Autodesk Inventor part; units mm, degrees
ref_plane "YZ Plane" through (0, 0, 0) normal (1, 0, 0) x (0, 1, 0)
ref_plane "XZ Plane" through (0, 0, 0) normal (0, 1, 0) x (-1, 0, 0)
ref_plane "XY Plane" through (0, 0, 0) normal (0, 0, 1) x (1, 0, 0)
sketch "Sketch1" plane through (0, 0, 0) normal (0, 1, 0) x (-1, 0, 0)
  line L0 (-3.8, -5.08) -> (100.076, -5.08)
  line L1 (100.076, -5.08) -> (100.076, 66.04)
  line L2 (100.076, 66.04) -> (-3.8, 66.04)
  line L3 (-3.8, 66.04) -> (-3.8, -5.08)
  circle A0 centre (11.176, 62.23) radius 1.75
  circle A1 centre (96.266, 62.23) radius 1.75
  circle A2 centre (96.266, 4.318) radius 1.75
  circle A3 centre (22.86, 4.318) radius 1.75
  line L4 (10.922, -14.9293) -> (10.922, -25.1011) construction
  point P0 (0, 0)
  dimension "d1" = 3.8
  dimension "d2" = 5.08
  dimension "d3" = 100.076
  dimension "d4" = 66.04
  dimension "d5" = 22.86
  dimension "d6" = 4.318
  dimension "d7" = 3.5
  dimension "d8" = 96.266
  dimension "d9" = 4.318
  dimension "d10" = 3.5
  dimension "d11" = 62.23
  dimension "d12" = 11.176
  dimension "d13" = 3.5
  dimension "d14" = 3.5
  dimension "d15" = 10.922
  dimension "d16" = 11.938
extrude "Extrusion1" add sketch "Sketch1" along normal blind 2
sketch "Sketch2" plane through (0, 2, 0) normal (0, 1, 0) x (1, 0, 0)
  circle A0 centre (-22.86, -4.318) radius 1.75
  line L0 (-16.922, 10.48) -> (-4.922, 10.48)
  line L1 (-4.922, 10.48) -> (-4.922, -4.318)
  line L2 (-4.922, -4.318) -> (-16.922, -4.318)
  line L3 (-16.922, -4.318) -> (-16.922, 10.48)
  line L4 (-10.922, -7.2674) -> (-10.922, -16.4399) construction
  line L5 (3.8, 5.08) -> (-100.076, 5.08)
  point P0 (0, 0)
  dimension "d20" = 11.938
  dimension "d21" = 6
  dimension "d22" = 12
  dimension "d25" = 5.4
extrude "Extrusion2" add sketch "Sketch2" along normal blind 12 contours L0 L1 L5 L3 | L5 L1 L2 L3
properties part number "printrboard"
Check sheet for the modelled part. Datum: model origin and axes. Units: mm. A direction names the side the tool comes from. Round coordinates to 2 decimals unless told otherwise and drop trailing zeros. Order: outer loops, then holes, each group sorted by start corner. A loop starts at its lowest first (then second) coordinate and runs counter-clockwise, first axis right, second up. Notation, with made-up numbers: (-18, 65) -> (-13, 65) arc R11 ccw to (-13, 74) -> close; hole circle Ø3 at (-24, 22.5). An arc over 180 degrees is marked (long way). One line per item, written item: value. Start each with the question number.
Q1. Mould release check, pull along Z, two halves, no side actions. Record for faces 5 (the face through (-11, 8, -10.48)), 6 (the face through (-11, 8, 4.318)), 7 (the face through (-94.518, 0.986, 4.241)), 8 (the face through (-100.076, 1, 30)): pulls with the +Z half, pulls with the -Z half, needs draft (parallel to the pull), parting line crosses it, or undercut.
Q2. Set-up check for faces 1 (the face through (-4.922, 8, -3)), 2 (the face through (-16.922, 8, -3)), 3 (the face through (-49, 1, 66.04)), 4 (the face through (-11, 2, -8)): record each of +Z, -Z, +X, -X, +Y, -Y from which the full face is reachable in a straight line by a thin tool's end or side.
Q3. Cross-section at A-A (x = -22.86). Record the boundary of the cut face in (y, z), and give its area (3 significant figures).
Q4. Gauge pin test, flat ends, axial feed: pin 1 Ø6 at (x, y) = (-22.5, 4) entering from -Z; pin 2 Ø4.5 at (x, z) = (-8, -8) entering from -Y; pin 3 Ø2 at (x, z) = (-11.176, 62.23) entering from +Y; pin 4 Ø8 at (x, z) = (-59.5, 56) entering from +Y. Record the tip position at first contact, or that the pin passes through.
Q5. Cross-section at C-C (z = -2.5). Record the boundary of the cut face in (x, y), and give its area (3 significant figures).
Q6. Cross-section at B-B (z = 62.23). Record the boundary of the cut face in (x, y).
Q7. Thickness scan on line 1 (Z direction, x = -22.86, y = 0.4); line 2 (Y direction, x = -85, z = 0); line 3 (Z direction, x = -13.5, y = 5.5). Record the ranges inside material, lowest first.
Q8. Cross-section at D-D (y = 4.25). Record the boundary of the cut face in (x, z), and give its area (3 significant figures).
Completed:
1. face 5: pulls with the -Z half
1. face 6: pulls with the +Z half
1. face 7: undercut
1. face 8: needs draft
2. face 1: +Z, -Z, +X, +Y
2. face 2: +Z, -Z, -X, +Y
2. face 3: +Z, +X, -X, +Y, -Y
2. face 4: -Z, +X, -X, -Y
3. outline: (0, -5.08) -> (2, -5.08) -> (2, 2.57) -> (0, 2.57) -> close; (0, 6.07) -> (2, 6.07) -> (2, 66.04) -> (0, 66.04) -> close
3. area: 135 mm²
4. pin 1: stops at z = -5.08
4. pin 2: stops at y = 2
4. pin 3: passes through
4. pin 4: stops at y = 2
5. outline: (-100.08, 0) -> (3.8, 0) -> (3.8, 2) -> (-4.92, 2) -> (-4.92, 14) -> (-16.92, 14) -> (-16.92, 2) -> (-100.08, 2) -> close
5. area: 352 mm²
6. outline: (-100.08, 0) -> (-98.02, 0) -> (-98.02, 2) -> (-100.08, 2) -> close; (-94.52, 0) -> (-12.93, 0) -> (-12.93, 2) -> (-94.52, 2) -> close; (-9.43, 0) -> (3.8, 0) -> (3.8, 2) -> (-9.43, 2) -> close
7. line 1: z = -5.08 to 2.57, 6.07 to 66.04
7. line 2: y = 0 to 2
7. line 3: z = -10.48 to 4.32
8. outline: (-16.92, -10.48) -> (-4.92, -10.48) -> (-4.92, 4.32) -> (-16.92, 4.32) -> close
8. area: 178 mm²
